Can you work these out from the model? Positions are in its coordinate system, mm. A direction names the side the tool comes from. Give positions to 0.01 mm unless a question says otherwise; leave off trailing zeros. Order: outer loops, then holes, each group sorted by start corner. A loop starts at its lowest first (then second) coordinate and runs counter-clockwise, first axis right, second up. Notation, with made-up numbers: M 44.25,68.25 L 57.25,68.25 A16 ccw 57.25,86.25 Z; hole C -18,-8.5 d8. An arc over 180 degrees is marked long. Use one line per item in the form item = value. Start each with the question number.
1. Will these pins go through, and if not, where does the flat tip stop? P1, Ø5, axis at y = -88.5, z = 5, coming from the -X side; P2, Ø5, axis at y = -88.5, z = 4, coming from the +X side.
2. I want a section at C-C, the plane z = 4.5. List the corners of the cut face in (x, y) for me, and give its area (3 significant figures).
3. We'd pull the mould along X, two halves only. Please class faces 4 (the face through (166, -63, 5)), 5 (the face through (-290, 11, 5)), 6 (the face through (190, 11, 5)), 7 (the face through (-251, -81, 5)): +X half, -X half, draft (parallel to the pull), parting line (faces both ways), or undercut.
4. I need wall thicknesses on L1, parallel to Y at x = 170, z = 4.75; L2, parallel to Y at x = 159, z = 8.5. Which ranges of each line are inside material? Lowest first, please.
5. For faces 1 (the face through (110, -93, 5)), 2 (the face through (-210, -93, 5)), 3 (the face through (-53, 1, 0)), which set-ups out of +Z, -Z, +X, -X, +Y, -Y let a thin tool reach every point of the face, with its end or its side?
6. I want a section at B-B, the plane x = 170. List the corners of the cut face in (y, z) for me.
7. I want a section at A-A, the plane y = -66. List the corners of the cut face in (x, z) for me.
```python
from build123d import *

# Parameters (mm, degrees)
ESQUISSE1_W             = 480
ESQUISSE1_H             = 210
BOSS_EXTRU_1_DEPTH      = 10
ESQUISSE2_W             = 80
ESQUISSE2_H             = 24
ENL_V_MAT_EXTRU_1_DEPTH = 11
ESQUISSE3_R             = 5
ENL_V_MAT_EXTRU_2_DEPTH = 11


with BuildPart() as part:
    # Esquisse1 → Boss.-Extru.1 (new body)
    with BuildSketch(Plane.XY):
        with Locations((-50, 0)):
            Rectangle(ESQUISSE1_W, ESQUISSE1_H)
    extrude(amount=BOSS_EXTRU_1_DEPTH)

    # Esquisse2 → Enlèv. mat.-Extru.1 (cut, through all)
    with BuildSketch(Plane.XY.offset(10)):
        with Locations((150, -93)):
            Rectangle(ESQUISSE2_W, ESQUISSE2_H)
        with Locations((-250, -93)):
            Rectangle(ESQUISSE2_W, ESQUISSE2_H)
    extrude(amount=-ENL_V_MAT_EXTRU_1_DEPTH, mode=Mode.SUBTRACT)

    # Esquisse3 → Enlèv. mat.-Extru.2 (cut, through all)
    with BuildSketch(Plane.XY.offset(10)):
        with Locations((170, -66)):
            Circle(ESQUISSE3_R)
    extrude(amount=-ENL_V_MAT_EXTRU_2_DEPTH, mode=Mode.SUBTRACT)


solid = part.part
```
Check result:
q1.P1 = -210
q1.P2 = 110
q2.outline = M -290,-81 L -210,-81 L -210,-105 L 110,-105 L 110,-81 L 190,-81 L 190,105 L -290,105 Z; hole C 170,-66 d10
q2.area = 96,900 mm2
q3.face_4 = undercut
q3.face_5 = -X half
q3.face_6 = +X half
q3.face_7 = draft
q4.L1 = -81 to -71, -61 to 105
q4.L2 = -81 to 105
q5.face_1 = +Z, -Z, +X, -Y
q5.face_2 = +Z, -Z, -X, -Y
q5.face_3 = -Z, +X, -X, +Y, -Y
q6.outline = M -81,0 L -71,0 L -71,10 L -81,10 Z; M -61,0 L 105,0 L 105,10 L -61,10 Z
q7.outline = M -290,0 L 165,0 L 165,10 L -290,10 Z; M 175,0 L 190,0 L 190,10 L 175,10 Z
